Can you work these out from the model? Positions are in its coordinate system, mm. Face numbers are marked on the shaded views. Coordinates: 2 decimals unless noted, no trailing zeros. Loops run counter-clockwise (first coordinate to the right, second up) from the corner with the lowest first, then second, coordinate; pieces in that order, holes last. Notation, with made-up numbers: M 18.5,2.5 L 54.5,2.5 A23 cw 54.5,11.5 Z; hole C 15,-8 d10. An arc over 180 degrees is marked long. Answer as a JSON object with one key per item and string values. Group by question number.
Item 1: If I drill on line 1 (Z direction, x = 46.75, y = 0); line 2 (Z direction, x = -24, y = 0); line 3 (X direction, y = 6.5, z = -14), over which ranges is the centre line in solid material (lowest first)?
Item 2: Suppose I cut it at D-D (y = -17.5). Write out the boundary of the cut face in (x, z), then the cut area to 3 significant figures.
Item 3: We'd pull the mould along X, two halves only. Please class the marked faces 1, 2 and 3: +X half, -X half, draft (parallel to the pull), parting line (faces both ways), or undercut.
Item 4: I'm going to push flat-ended pins straight in: pin 1 Ø5 at (x, z) = (27, -8) entering from +Y; pin 2 Ø16 at (x, z) = (0.5, -7) entering from -Y; pin 3 Ø2 at (x, y) = (-4, -19) entering from +Z. Where does each tip first touch, or does it pass through?
Item 5: Suppose I cut it at B-B (y = 5.5). Write out the boundary of the cut face in (x, z).
Item 6: Suppose I cut it at A-A (z = 0). Write out the boundary of the cut face in (x, y), then the cut area to 3 significant figures.
Item 7: Suppose I cut it at C-C (x = -27). Write out the boundary of the cut face in (y, z).
```python
from build123d import *

# Parameters (mm, degrees)
F0_R      = 19.05
F2_DEPTH  = 50
F1_R      = 19.05
F4_DEPTH  = 35
F3_R      = 14.3508300954
F5_DEPTH  = 100.001
F6_R      = 14.05
F7_DEPTH  = 32.078017988
F8_R      = 16.05
F9_DEPTH  = 5
F10_R     = 16.3508300954
F11_DEPTH = 5
F12_R     = 16.3508300954
F13_DEPTH = 5


with BuildPart() as f2:
    # F0 (on Right) → F2 (new body, symmetric)
    with BuildSketch(Plane.YZ):
        Circle(F0_R)
    extrude(amount=F2_DEPTH, both=True)

    # F1 (on Front) → F4 (join)
    with BuildSketch(Plane.XZ):
        Circle(F1_R)
    extrude(amount=F4_DEPTH)

    # F3 (on face) → F5 (cut, through all)
    with BuildSketch(Plane.YZ.offset(50)):
        Circle(F3_R)
    extrude(amount=-F5_DEPTH, mode=Mode.SUBTRACT)

    # F6 (on face) → F7 (cut, through all)
    with BuildSketch(Plane.XZ.offset(35)):
        Circle(F6_R)
    extrude(amount=-F7_DEPTH, mode=Mode.SUBTRACT)

    # F8 (on face) → F9 (cut)
    with BuildSketch(Plane.XZ.offset(35)):
        Circle(F8_R)
    extrude(amount=-F9_DEPTH, mode=Mode.SUBTRACT)

    # F10 (on face) → F11 (cut)
    with BuildSketch(Plane.YZ.offset(50)):
        Circle(F10_R)
    extrude(amount=-F11_DEPTH, mode=Mode.SUBTRACT)

    # F12 (on face) → F13 (cut)
    with BuildSketch(Plane(origin=(-50, 0, 0), x_dir=(0, -1, 0), z_dir=(-1, 0, 0))):
        Circle(F12_R)
    extrude(amount=-F13_DEPTH, mode=Mode.SUBTRACT)


solid = f2.part
```
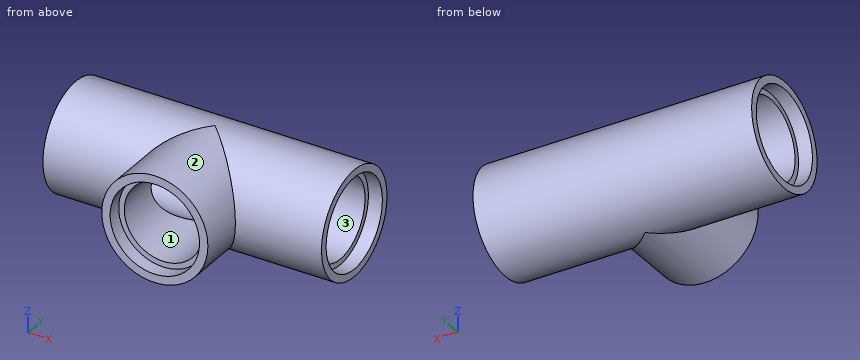
From the geometry:
{
 "1": {"line 1": "-19.05 to -16.35, 16.35 to 19.05", "line 2": "-19.05 to -14.35, 14.35 to 19.05", "line 3": "-45 to 45"},
 "2": {"outline": "M -50,-7.53 L -17.5,-7.53 A19.05 ccw 17.5,-7.53 L 50,-7.53 L 50,7.53 L 17.5,7.53 A19.05 ccw -17.5,7.53 L -50,7.53 Z; hole C 0,0 d28.1", "area": "1,470 mm2"},
 "3": {"face 1": "undercut", "face 2": "parting line", "face 3": "draft"},
 "4": {"pin 1": "y = 18.24", "pin 2": "y = -30", "pin 3": "z = 18.81"},
 "5": {"outline": "M -50,-18.24 L 50,-18.24 L 50,-15.4 L 45,-15.4 L 45,-13.26 L -45,-13.26 L -45,-15.4 L -50,-15.4 Z; M -50,15.4 L -45,15.4 L -45,13.26 L 45,13.26 L 45,15.4 L 50,15.4 L 50,18.24 L -50,18.24 Z"},
 "6": {"outline": "M -50,-19.05 L -19.05,-19.05 L -19.05,-35 L -16.05,-35 L -16.05,-30 L -14.05,-30 L -14.05,-14.35 L -45,-14.35 L -45,-16.35 L -50,-16.35 Z; M -50,16.35 L -45,16.35 L -45,14.35 L 45,14.35 L 45,16.35 L 50,16.35 L 50,19.05 L -50,19.05 Z; M 14.05,-30 L 16.05,-30 L 16.05,-35 L 19.05,-35 L 19.05,-19.05 L 50,-19.05 L 50,-16.35 L 45,-16.35 L 45,-14.35 L 14.05,-14.35 Z", "area": "907 mm2"},
 "7": {"outline": "C 0,0 d38.1; hole C 0,0 d28.7"}
}
